```python
from build123d import *

# Parameters (mm, degrees)
F0_W     = 103.2
F0_H     = 153.2
F0_W_2   = 100
F0_H_2   = 150
F1_DEPTH = 24
F2_W     = 100
F2_H     = 150
F3_DEPTH = 3.2
F4_W     = 103.2
F4_H     = 2.6
F5_DEPTH = 30


with BuildPart() as f1:
    # F0 (on Top) → F1 (new body)
    with BuildSketch(Plane.XY):
        Rectangle(F0_W, F0_H)
        Rectangle(F0_W_2, F0_H_2, mode=Mode.SUBTRACT)
    extrude(amount=F1_DEPTH)

    # F2 (on Top) → F3 (join)
    with BuildSketch(Plane.XY):
        Rectangle(F2_W, F2_H)
    extrude(amount=F3_DEPTH)

    # F4 (on Top) → F5 (join)
    with BuildSketch(Plane.XY):
        with Locations((0, 75.3)):
            Rectangle(F4_W, F4_H)
    extrude(amount=F5_DEPTH)


solid = f1.part
```
Here's how the part is built. I have some questions about the finished solid (model axes, mm). A direction names the side the tool comes from. Round coordinates to 2 decimals unless told otherwise and drop trailing zeros. Write each loop counter-clockwise with the first axis right and the second up, starting at its lowest first coordinate (ties: lowest second). Pieces come first, ordered by that corner, then holes. Notation, with made-up numbers: M 40.25,34 L 63.25,34 A28 cw 63.25,68 Z; hole C 51,-28 d2. An arc over 180 degrees is marked long. Answer as CSV lines item,"result". Start each with the question number.
1. Suppose I cut it at C-C on y = -33.5. Write out the boundary of the cut face in (x, z).
2. I'm going to push a flat-ended pin straight in: pin 1 Ø4 at (x, y) = (27.5, 47) entering from +Z. Where does the tip first touch, or does it pass through?
3. Suppose I cut it at A-A on z = 5. Write out the boundary of the cut face in (x, y), then the cut area to 3 significant figures.
4. Suppose I cut it at B-B on x = 19.5. Write out the boundary of the cut face in (y, z), then the cut area to 3 significant figures.
5. I need wall thicknesses on probe 1 along Y at (x, z) = (-15.5, 19.75); probe 2 along X at (y, z) = (54, 20.5); probe 3 along Z at (x, y) = (-0.5, -25.5). Which ranges of each line are inside material? Lowest first, please.
6. Thinking about a two-plate mould opening in X: for faces 3 (the flat face through (-1, 76.6, 15)), 4 (the flat face through (-51.6, -1, 11)), 5 (the flat face through (-50, -2, 13)), which applies, released by +X, released by -X, zero draft, split by the parting line, or undercut?
7. On a 3-axis mill with a long thin cutter (end or side, diameter ignored), from which of +Z, -Z, +X, -X, +Y, -Y can I reach the whole of each face in a straight line? I mean faces 1 (the flat face through (51.6, -1, 11)), 2 (the flat face through (-1, -75, 13)). Say none if no direction works.
Check result:
1,outline,"M -51.6,0 L 51.6,0 L 51.6,24 L 50,24 L 50,3.2 L -50,3.2 L -50,24 L -51.6,24 Z"
2,pin 1,"stops at z = 3.2"
3,outline,"M -51.6,-76.6 L 51.6,-76.6 L 51.6,76.6 L -51.6,76.6 Z; hole M -50,-75 L 50,-75 L 50,74 L -50,74 Z"
3,area,"910 mm2"
4,outline,"M -76.6,0 L 76.6,0 L 76.6,30 L 74,30 L 74,3.2 L -75,3.2 L -75,24 L -76.6,24 Z"
4,area,"593 mm2"
5,probe 1,"y = -76.6 to -75, 74 to 76.6"
5,probe 2,"x = -51.6 to -50, 50 to 51.6"
5,probe 3,"z = 0 to 3.2"
6,face 3,"zero draft"
6,face 4,"released by -X"
6,face 5,"undercut"
7,face 1,"+Z, -Z, +X, +Y, -Y"
7,face 2,"+Z"
